Design review of the part built by this model. Coordinates are the model's own, in mm. Face numbers are marked on the shaded views. A direction names the side the tool comes from. Coordinates: 2 decimals unless noted, no trailing zeros. Write each loop counter-clockwise with the first axis right and the second up, starting at its lowest first coordinate (ties: lowest second). Pieces come first, ordered by that corner, then holes. Notation, with made-up numbers: (61, -18) - (111, -18) arc R25 ccw to (111, 19) - close; hole circle Ø1 at (68, 21). An arc over 180 degrees is marked (long way). Use a Markdown table: item, result.
from build123d import *

# Parameters (mm, degrees)
FILLET1_R          = 2
CUT_EXTRUDE1_START = 34
CUT_EXTRUDE1_DEPTH = 10
CUT_EXTRUDE2_START = 26.5
CUT_EXTRUDE2_DEPTH = 10


with BuildPart() as part:
    # Sketch1 → Revolve1 (revolve)
    with BuildSketch(Plane(origin=(0, 0, 0), x_dir=(0, 0, -1), z_dir=(1, 0, 0))):
        Polygon((0, 0), (-365.5, 0), (-365.5, 30), (-297.5, 30), (-297.5, 32.5), (-167.5, 32.5), (-167.5, 50), (-138.5, 50), (-138.5, 40), (-58.5, 40), (-58.5, 30), (0, 30), align=None)
    revolve(axis=Axis((0, 0, 0), (0, 0, -1)))

    # Fillet1
    fillet1_edges = [part.edges().sort_by_distance(p)[0] for p in [
        (0, -30, 365.5),
        (0, -30, 0),
    ]]
    fillet(fillet1_edges, radius=FILLET1_R)

    # Sketch2 → Cut-Extrude1 (cut)
    with BuildSketch(Plane(origin=(0, 0, 0), x_dir=(1, 0, 0), z_dir=(0, 1, 0)).offset(CUT_EXTRUDE1_START)):
        with BuildLine():
            Line((8, -71.5), (8, -125.5))
            ThreePointArc((8, -125.5), (0, -133.5), (-8, -125.5))
            Line((-8, -125.5), (-8, -71.5))
            ThreePointArc((-8, -71.5), (0, -63.5), (8, -71.5))
        make_face()
    extrude(amount=CUT_EXTRUDE1_DEPTH, mode=Mode.SUBTRACT)

    # Sketch3 → Cut-Extrude2 (cut)
    with BuildSketch(Plane(origin=(0, 0, 0), x_dir=(1, 0, 0), z_dir=(0, 1, 0)).offset(CUT_EXTRUDE2_START)):
        with BuildLine():
            Line((6, -176), (6, -289))
            ThreePointArc((6, -289), (0, -295), (-6, -289))
            Line((-6, -289), (-6, -176))
            ThreePointArc((-6, -176), (0, -170), (6, -176))
        make_face()
    extrude(amount=CUT_EXTRUDE2_DEPTH, mode=Mode.SUBTRACT)


solid = part.part
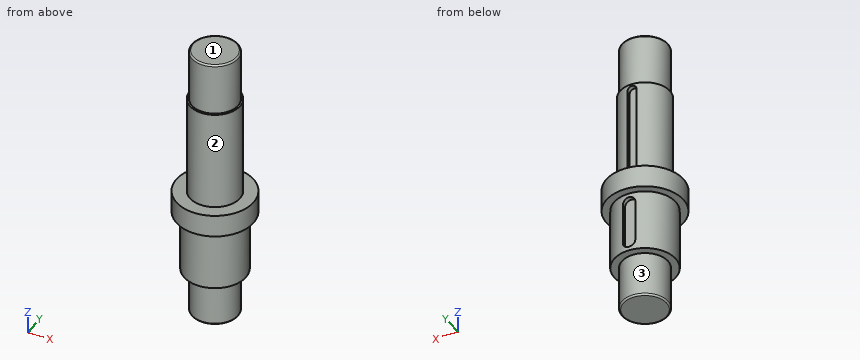
(1) Take a section at C-C on z = 222. Write out the cut boundary in (x, y).
Determined:
| item | result |
|---|---|
| outline | (-6, 26.5) - (-6, 31.94) arc R32.5 ccw (long way) to (6, 31.94) - (6, 26.5) - close |
(2) Machinability: for the marked faces 1, 2 and 3, which of the approach directions +Z, -Z, +X, -X, +Y, -Y give a long, thin tool a straight path to every point of the face, cutting with its end or side? Answer none if there is none.
Determined:
| item | result |
|---|---|
| face 1 | +Z, +X, -X, +Y, -Y |
| face 2 | +Z |
| face 3 | -Z |
(3) Take a section at B-B on z = 149. Write out the cut boundary in (x, y), and give its area (3 significant figures).
Determined:
| item | result |
|---|---|
| outline | circle Ø100 at (0, 0) |
| area | 7,850 mm2 |
(4) For L1, parallel to Z at x = -38, y = -8; L2, parallel to Z at x = -4, y = 39.5; L3, parallel to Z at x = 32.5, y = -24, list the stretches that pass through material, from the lowest coordinate up. Write a range as from..to.
Determined:
| item | result |
|---|---|
| L1 | 58.5..167.5 |
| L2 | 58.5..64.57, 132.43..167.5 |
| L3 | 138.5..167.5 |
(5) For pin 1 (10 mm diameter, centred on x = 31, y = 25, fed in from +Z); pin 2 (12 mm diameter, centred on x = 9, z = 269, fed in from -Y); pin 3 (3 mm diameter, centred on x = -21.5, y = -24.5, fed in from -Z); pin 4 (24 mm diameter, centred on x = -16.5, y = -8.5, fed in from -Z), all flat-tipped, find the tip position at first contact; note any pin that passes through.
Determined:
| item | result |
|---|---|
| pin 1 | z = 167.5 |
| pin 2 | y = -32.36 |
| pin 3 | z = 58.5 |
| pin 4 | z = 0 |
(6) Take a section at A-A on y = 0. Write out the cut boundary in (x, z).
Determined:
| item | result |
|---|---|
| outline | (-50, 138.5) - (-40, 138.5) - (-40, 58.5) - (-30, 58.5) - (-30, 2) arc R2 ccw to (-28, 0) - (28, 0) arc R2 ccw to (30, 2) - (30, 58.5) - (40, 58.5) - (40, 138.5) - (50, 138.5) - (50, 167.5) - (32.5, 167.5) - (32.5, 297.5) - (30, 297.5) - (30, 363.5) arc R2 ccw to (28, 365.5) - (-28, 365.5) arc R2 ccw to (-30, 363.5) - (-30, 297.5) - (-32.5, 297.5) - (-32.5, 167.5) - (-50, 167.5) - close |
